```python
from build123d import *

# Parameters (mm, degrees)
SKETCH1_W           = 11.5
SKETCH1_H           = 23
BOSS_EXTRUDE1_DEPTH = 11
SKETCH3_W           = 11.5
SKETCH3_H           = 23
BOSS_EXTRUDE3_DEPTH = 6
SKETCH4_W           = 9.5
SKETCH4_H           = 6
CUT_EXTRUDE1_DEPTH  = 27.135464411
SKETCH7_W           = 2
SKETCH7_H           = 6
CUT_EXTRUDE2_DEPTH  = 10
SKETCH8_W           = 11.5
SKETCH8_H           = 23
BOSS_EXTRUDE4_DEPTH = 4
SKETCH9_W           = 19
SKETCH9_H           = 5
CUT_EXTRUDE3_DEPTH  = 23.12464689
FILLET1_R           = 5


with BuildPart() as part:
    # Sketch1 → Boss-Extrude1 (new body)
    with BuildSketch(Plane(origin=(0, 0, 0), x_dir=(1, 0, 0), z_dir=(0, 1, 0))):
        Rectangle(SKETCH1_W, SKETCH1_H)
    extrude(amount=BOSS_EXTRUDE1_DEPTH)

    # Sketch3 → Boss-Extrude3 (add)
    with BuildSketch(Plane.XZ):
        Rectangle(SKETCH3_W, SKETCH3_H)
    extrude(amount=BOSS_EXTRUDE3_DEPTH)

    # Sketch4 → Cut-Extrude1 (cut, through all)
    with BuildSketch(Plane.XY.offset(11.5)):
        with Locations((0, -3)):
            Rectangle(SKETCH4_W, SKETCH4_H)
    extrude(amount=-CUT_EXTRUDE1_DEPTH, mode=Mode.SUBTRACT)

    # Sketch7 → Cut-Extrude2 (cut)
    with BuildSketch(Plane.XZ):
        Rectangle(SKETCH7_W, SKETCH7_H)
    extrude(amount=-CUT_EXTRUDE2_DEPTH, mode=Mode.SUBTRACT)

    # Sketch8 → Boss-Extrude4 (add)
    with BuildSketch(Plane(origin=(0, 11, 0), x_dir=(1, 0, 0), z_dir=(0, 1, 0))):
        Rectangle(SKETCH8_W, SKETCH8_H)
    extrude(amount=BOSS_EXTRUDE4_DEPTH)

    # Sketch9 → Cut-Extrude3 (cut, through all)
    with BuildSketch(Plane.ZY.offset(5.75)):
        with Locations((0, 12.5)):
            Rectangle(SKETCH9_W, SKETCH9_H)
    extrude(amount=-CUT_EXTRUDE3_DEPTH, mode=Mode.SUBTRACT)

    # Fillet1
    fillet1_edges = [part.edges().sort_by_distance(p)[0] for p in [
        (0, 10, -9.5),
        (0, 10, 9.5),
    ]]
    fillet(fillet1_edges, radius=FILLET1_R - 0.0001)  # a hair under: the kernel refuses the full size


solid = part.part
```
For this review, take the finished solid that the model builds, in its own axes (mm). A direction names the side the tool comes from. Give positions to 0.01 mm unless a question says otherwise; leave off trailing zeros. Write each loop counter-clockwise with the first axis right and the second up, starting at its lowest first coordinate (ties: lowest second). Pieces come first, ordered by that corner, then holes.
Item 1: Take a section at B-B (z = 0.5). Give the boundary of the cut face in (x, y), and give its area (3 significant figures).
Item 2: Insertion check: P1, Ø1.5, axis at x = 0.5, z = -8, coming from the -Y side; P2, Ø1.5, axis at x = -1.5, y = -2.5, coming from the -Z side; P3, Ø4, axis at x = -4.5, z = 6.5, coming from the +Y side. Each pin has a flat end and moves straight along its axis. Give the tip position at first contact, or say it passes through.
Item 3: The part is to be moulded in two halves that separate along Z. For faces 1 (the face through (0, 7, 11.5)), 2 (the face through (1.2, 10, -0.1)), 3 (the face through (5.75, 2, 0)), say which applies: +Z half, -Z half, draft (parallel to the pull), parting line (faces both ways), or undercut.
Item 4: Take a section at A-A (y = -2). Give the boundary of the cut face in (x, z).
Item 5: Take a section at D-D (y = 4.25). Give the boundary of the cut face in (x, z).
Item 6: Wall thickness on probe 1 along X at (y, z) = (3, 0.5); probe 2 along X at (y, z) = (-0.25, -2.5); probe 3 along Y at (x, z) = (0.5, -4.75): over which ranges is each line inside the solid? List them lowest first.
Item 7: Machinability: for faces 4 (the face through (0, 5, -3)), 5 (the face through (-4.75, -3, 0)), 6 (the face through (0.08, 11.5, -8.07)), 7 (the face through (0, 15, 10)), which of the approach directions +Z, -Z, +X, -X, +Y, -Y give a long, thin tool a straight path to every point of the face, cutting with its end or side? Answer none if there is none.
Established:
1. outline: (-5.75, -6) - (-4.75, -6) - (-4.75, 0) - (-1, 0) - (-1, 10) - (-5.75, 10) - close; (1, 0) - (4.75, 0) - (4.75, -6) - (5.75, -6) - (5.75, 10) - (1, 10) - close
1. area: 107 mm2
2. P1: stops at y = 0
2. P2: passes through
2. P3: stops at y = 12
3. face 1: +Z half
3. face 2: undercut
3. face 3: draft
4. outline: (-5.75, -11.5) - (-4.75, -11.5) - (-4.75, 11.5) - (-5.75, 11.5) - close; (4.75, -11.5) - (5.75, -11.5) - (5.75, 11.5) - (4.75, 11.5) - close
5. outline: (-5.75, -11.5) - (5.75, -11.5) - (5.75, 11.5) - (-5.75, 11.5) - close; hole (-1, -3) - (1, -3) - (1, 3) - (-1, 3) - close
6. probe 1: x = -5.75 to -1, 1 to 5.75
6. probe 2: x = -5.75 to -4.75, 4.75 to 5.75
6. probe 3: y = 0 to 10.01
7. face 4: +Y, -Y
7. face 5: +Z, -Z, -Y
7. face 6: +X, -X, +Y
7. face 7: +Z, -Z, +X, -X, +Y
